Could you check a few things on this model? Use its own coordinates, in mm. Coordinates: 2 decimals unless noted, no trailing zeros. Loops run counter-clockwise (first coordinate to the right, second up) from the corner with the lowest first, then second, coordinate; pieces in that order, holes last.
1) Imagine slicing it at D-D on x = 40. Please give me the cut outline in (y, z).
2) Imagine slicing it at B-B on z = 16. Please give me the cut outline in (x, y).
3) Thinking about a two-plate mould opening in X: for faces 1 (the face through (27, 0, 20)), 2 (the face through (35, 0, 10)), 3 (the face through (23.49, -14.59, 9.86)), which applies, released by +X, released by -X, zero draft, split by the parting line, or undercut?
4) Imagine slicing it at A-A on x = 0. Please give me the cut outline in (y, z).
5) Imagine slicing it at C-C on y = -3. Please give me the cut outline in (x, z), plus the area to 3 significant figures.
6) Will these pins go through, and if not, where does the flat tip stop? P1, Ø6, axis at y = -5, z = 10, coming from the -X side; P2, Ø6, axis at x = -10.5, z = 15.5, coming from the +Y side; P3, Ø21.5, axis at x = 0, y = 0, coming from the -Z side; P4, Ø5, axis at x = 9, z = 3.5, coming from the +Y side.
7) If I drill on line 1 along Y through (x, z) = (0, 20.25); line 2 along Z through (x, y) = (45, -1.5); line 3 along Y through (x, z) = (8.5, 2.5), over which ranges is the centre line in solid material (lowest first)?
```python
from build123d import *

# Parameters (mm, degrees)
F0_R     = 5
F1_DEPTH = 15
F0_R_2   = 12
F2_DEPTH = 30
F3_DEPTH = 20


with BuildPart() as f1:
    # F0 (on Top) → F1 (new body)
    with BuildSketch(Plane.XY):
        with BuildLine():
            ThreePointArc((5, 19.364917), (15.811388, 12.247449), (20, 0))
            ThreePointArc((20, 0), (15.811388, -12.247449), (5, -19.364917))
            Line((5, -19.364917), (42.5, -9.682458))
            ThreePointArc((42.5, -9.682458), (50, 0), (42.5, 9.682458))
            Line((42.5, 9.682458), (5, 19.364917))
        make_face()
        with Locations((40, 0)):
            Circle(F0_R, mode=Mode.SUBTRACT)
    extrude(amount=F1_DEPTH)

    # F0 (on Top) → F2 (join)
    with BuildSketch(Plane.XY):
        with BuildLine():
            ThreePointArc((5, -19.364917), (15.811388, -12.247449), (20, 0))
            ThreePointArc((20, 0), (15.811388, 12.247449), (5, 19.364917))
            ThreePointArc((5, 19.364917), (-20, 0), (5, -19.364917))
        make_face()
        Circle(F0_R_2, mode=Mode.SUBTRACT)
    extrude(amount=F2_DEPTH)

    # F0 (on Top) → F3 (join)
    with BuildSketch(Plane.XY):
        with BuildLine():
            ThreePointArc((5, 19.364917), (15.811388, 12.247449), (20, 0))
            ThreePointArc((20, 0), (15.811388, -12.247449), (5, -19.364917))
            Line((5, -19.364917), (42.5, -9.682458))
            ThreePointArc((42.5, -9.682458), (50, 0), (42.5, 9.682458))
            Line((42.5, 9.682458), (5, 19.364917))
        make_face()
        with Locations((40, 0)):
            Circle(F0_R, mode=Mode.SUBTRACT)
    extrude(amount=F3_DEPTH)


solid = f1.part
```
Filled in:
1. outline: (-10.33, 0) - (-5, 0) - (-5, 20) - (-10.33, 20) - close; (5, 0) - (10.33, 0) - (10.33, 20) - (5, 20) - close
2. outline: (5, -19.36) - (42.5, -9.68) arc R10 ccw to (42.5, 9.68) - (5, 19.36) arc R20 ccw (long way) to start; hole circle Ø24 at (0, 0); hole circle Ø10 at (40, 0)
3. face 1: zero draft
3. face 2: undercut
3. face 3: released by +X
4. outline: (-20, 0) - (-12, 0) - (-12, 30) - (-20, 30) - close; (12, 0) - (20, 0) - (20, 30) - (12, 30) - close
5. outline: (-19.77, 0) - (-11.62, 0) - (-11.62, 30) - (-19.77, 30) - close; (11.62, 0) - (36, 0) - (36, 20) - (19.77, 20) - (19.77, 30) - (11.62, 30) - close; (44, 0) - (49.54, 0) - (49.54, 20) - (44, 20) - close
5. area: 925 mm2
6. P1: stops at x = -19.9
6. P2: stops at y = 18.54
6. P3: passes through
6. P4: stops at y = 18.98
7. line 1: y = -20 to -12, 12 to 20
7. line 2: z = 0 to 20
7. line 3: y = -18.46 to -8.47, 8.47 to 18.46
